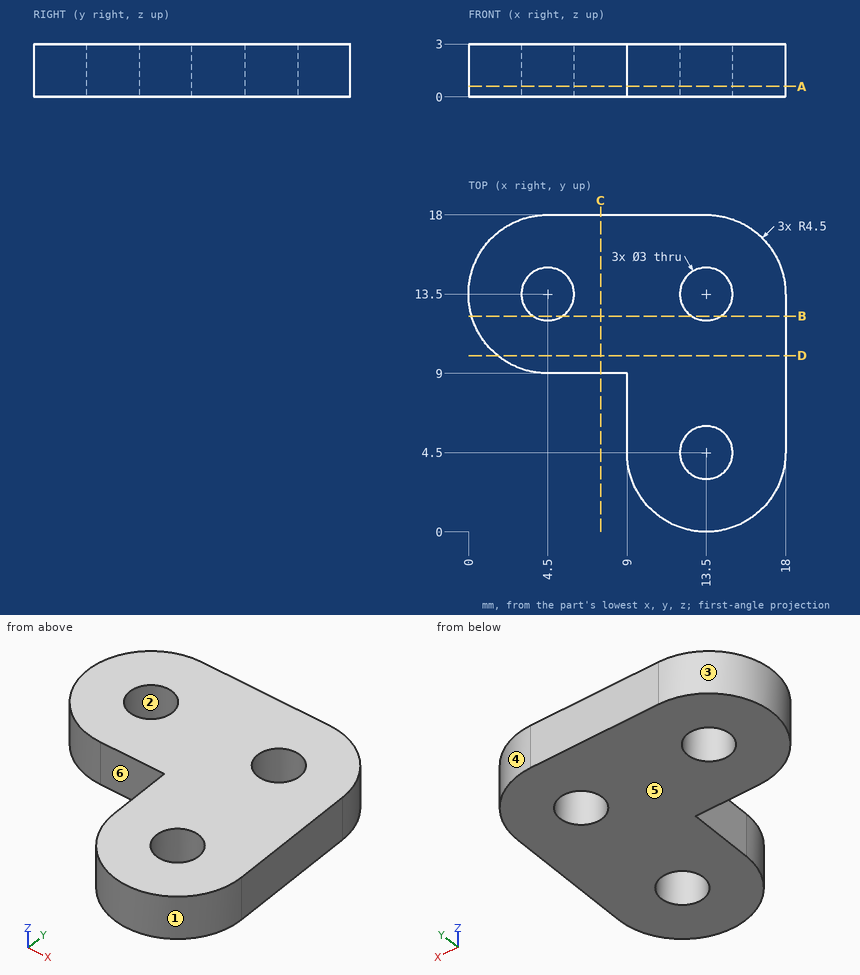
Could you check a few things on this drawing? It's one solid part, dimensions in mm from its lowest x, y, z. A direction names the side the tool comes from. Give positions to 0.01 mm unless a question says otherwise; leave off trailing zeros. Order: outer loops, then holes, each group sorted by start corner. A loop starts at its lowest first (then second) coordinate and runs counter-clockwise, first axis right, second up. Notation, with made-up numbers: (60, 15.5) - (69, 15.5) arc R32 cw to (69, 53.5) - close; hole circle Ø4 at (9.25, 37). An arc over 180 degrees is marked (long way). Answer as a JSON object with one key per item and string values. Group by question number.
Item 1: If we section it at D-D on y = 10: Please give me the cut outline in (x, z).
Item 2: For P1, Ø1.5, axis at y = 6, z = 2, coming from the -X side; P2, Ø6, axis at x = 8, y = 14, coming from the -Z side; P3, Ø0.9, axis at x = 6.5, z = 1.5, coming from the -Y side, each with a flat end and sliding along its axis, tell me the tip position at first contact or that it passes through.
Item 3: If we section it at B-B on y = 12.25: Please give me the cut outline in (x, z), and give its area (3 significant figures).
Item 4: If we section it at C-C on x = 7.5: Please give me the cut outline in (y, z), and give its area (3 significant figures).
Item 5: If we mould it in two halves opening along Y, with no side actions, what happens to the marked faces 1, 2, 3 and 4? For each: pulls with the +Y half, pulls with the -Y half, needs draft (parallel to the pull), parting line crosses it, or undercut.
Item 6: If we section it at A-A on z = 0.6: Please give me the cut outline in (x, y).
Item 7: Which directions (+Z, -Z, +X, -X, +Y, -Y) give clear straight access to the entire face, cutting with the end or side of a thin tool? Please do the marked faces 5 and 6.
Item 8: Please list where these lines run through material, in increasing order: probe 1 along X at (y, z) = (13.5, 1.95); probe 2 along Y at (x, z) = (14.25, 1.75).
Result set:
{
 "1": {"outline": "(1.67, 0) - (18, 0) - (18, 3) - (1.67, 3) - close"},
 "2": {"P1": "x = 9", "P2": "z = 0", "P3": "y = 9"},
 "3": {"outline": "(0.18, 0) - (3.67, 0) - (3.67, 3) - (0.18, 3) - close; (5.33, 0) - (12.67, 0) - (12.67, 3) - (5.33, 3) - close; (14.33, 0) - (18, 0) - (18, 3) - (14.33, 3) - close", "area": "43.5 mm²"},
 "4": {"outline": "(9, 0) - (18, 0) - (18, 3) - (9, 3) - close", "area": "27.0 mm²"},
 "5": {"face 1": "pulls with the -Y half", "face 2": "undercut", "face 3": "parting line crosses it", "face 4": "pulls with the +Y half"},
 "6": {"outline": "(4.5, 9) - (9, 9) - (9, 4.5) arc R4.5 ccw to (18, 4.5) - (18, 13.5) arc R4.5 ccw to (13.5, 18) - (4.5, 18) arc R4.5 ccw to start; hole circle Ø3 at (4.5, 13.5); hole circle Ø3 at (13.5, 4.5); hole circle Ø3 at (13.5, 13.5)"},
 "7": {"face 5": "-Z, +X, -X, +Y, -Y", "face 6": "+Z, -Z, -X, -Y"},
 "8": {"probe 1": "0 to 3, 6 to 12, 15 to 18", "probe 2": "0.06 to 3.2, 5.8 to 12.2, 14.8 to 17.94"}
}
